```python
from build123d import *

# Parameters (mm, degrees)
BOSS_EXTRUDE1_DEPTH      = 5
BOSS_EXTRUDE1_DEPTH_BACK = 13
SKETCH2_R                = 1.5
CUT_EXTRUDE1_DEPTH       = 66.915554427
SKETCH4_W                = 8
SKETCH4_H                = 4.7
BOSS_EXTRUDE2_DEPTH      = 6
CUT_EXTRUDE3_START       = -5
CUT_EXTRUDE3_DEPTH       = 61.915554427
CUT_EXTRUDE4_DEPTH       = 68.080998169
CHAMFER1_SIZE            = 2.5


with BuildPart() as part:
    # Sketch1 → Boss-Extrude1 (new, two sides: drawn at the far end of the back side and taken through both)
    with BuildSketch(Plane.XY.offset(-BOSS_EXTRUDE1_DEPTH_BACK)):
        Polygon((0, 6), (5, 6), (5, -5), (-20.67950334, -22.556349186), (-49.056349186, -22.556349186), (-60.556349186, -11.056349186), (-46.414213562, 3.085786438), (-34.328427125, -9), (-21.164213562, -9), (-8, 0), (0, 0), align=None)
    extrude(amount=BOSS_EXTRUDE1_DEPTH + BOSS_EXTRUDE1_DEPTH_BACK)

    # Sketch2 → Cut-Extrude1 (cut, through all)
    with BuildSketch(Plane(origin=(0, 0, 0), x_dir=(1, 0, 0), z_dir=(0, 1, 0))):
        with Locations(Location((-3, 3.95, 0), (0, 0, 270))):
            Circle(SKETCH2_R)
    extrude(amount=-CUT_EXTRUDE1_DEPTH, mode=Mode.SUBTRACT)

    # Sketch4 → Boss-Extrude2 (add)
    with BuildSketch(Plane(origin=(0, 0, 0), x_dir=(1, 0, 0), z_dir=(0, 1, 0))):
        with Locations((-4, -2.65)):
            Rectangle(SKETCH4_W, SKETCH4_H)
        with Locations((-4, 10.65)):
            Rectangle(SKETCH4_W, SKETCH4_H)
    extrude(amount=BOSS_EXTRUDE2_DEPTH)

    # Sketch5 → Cut-Extrude3 (cut, through all)
    with BuildSketch(Plane(origin=(0, 0, 0), x_dir=(1, 0, 0), z_dir=(0, 1, 0)).offset(CUT_EXTRUDE3_START)):
        Polygon((-1.267949192, 0.95), (-4.732050808, 0.95), (-6.464101615, 3.95), (-4.732050808, 6.95), (-1.267949192, 6.95), (0.464101615, 3.95), align=None)
    extrude(amount=-CUT_EXTRUDE3_DEPTH, mode=Mode.SUBTRACT)

    # Sketch6 → Cut-Extrude4 (cut, through all)
    with BuildSketch(Plane.XY.offset(5)):
        Polygon((-42.85, -22.556349186), (-49.056349186, -22.556349186), (-60.556349186, -11.056349186), (-46.414213562, 3.085786438), (-34.328427125, -9), (-42.85, -9), align=None)
    extrude(amount=-CUT_EXTRUDE4_DEPTH, mode=Mode.SUBTRACT)

    # Sketch7 → Cut-Revolve1 (revolve, cut)
    with BuildSketch(Plane.XY.offset(-3.95), mode=Mode.PRIVATE) as cut_revolve1_sk:
        Polygon((-24.85, -15.1), (-25.85, -15.1), (-45.997007673, -15.1), (-45.997007673, -12), (-39.790264322, -12), (-38.290264322, -12.35), (-25.85, -12.35), (-24.85, -12.85), align=None)
    revolve(cut_revolve1_sk.sketch.rotate(Axis((-45.997007673, -15.1, -3.95), (1, 0, 0)), 180), axis=Axis((-45.997007673, -15.1, -3.95), (1, 0, 0)), mode=Mode.SUBTRACT)

    # Chamfer1
    chamfer1_edges = [part.edges().sort_by_distance(p)[0] for p in [
        (-42.85, -9, -4),
    ]]
    chamfer(chamfer1_edges, length=CHAMFER1_SIZE)


solid = part.part
```
The model under review builds one solid part; all positions refer to its coordinate system, in mm. A direction names the side the tool comes from. Round coordinates to 2 decimals unless told otherwise and drop trailing zeros. Loops run counter-clockwise (first coordinate to the right, second up) from the corner with the lowest first, then second, coordinate; pieces in that order, holes last. Notation, with made-up numbers: M -14.5,27.5 L 16.5,27.5 A23 cw 16.5,42.5 Z; hole C 13,4 d2. An arc over 180 degrees is marked long. Put each result on its own line as item: value.
Q1. To check wall thickness, follow L1, parallel to Z at x = -41.4, y = -15.1; L2, parallel to Z at x = -1, y = 0.25; L3, parallel to Y at x = -39.5, z = 2.25. State the ranges of each line that lie inside material, in increasing order.
Result set:
L1: z = -13 to -7.05, -0.85 to 5
L2: z = -13 to -8.3, 0.3 to 5
L3: y = -22.56 to -9
Q2. Mouldability with a two-part tool opening along Y and no side actions: class faces 6 (the cylindrical face through (-41.3, -12.82, -6.05)), 7 (the flat face through (-5, 0, -4)), 8 (the flat face through (-5.586, -8.864, -2.429)), 9 (the cylindrical face through (-31.98, -17.64, -2.9)) as released by +Y, released by -Y, zero draft, split by the parting line, or undercut.
Result set:
face 6: undercut
face 7: released by +Y
face 8: zero draft
face 9: undercut
Q3. Consider section C-C, the plane y = -15.1. Give the boundary of the cut face in (x, z).
Result set:
outline: M -42.85,-13 L -9.77,-13 L -9.77,5 L -42.85,5 L -42.85,-0.85 L -39.79,-0.85 L -38.29,-1.2 L -25.85,-1.2 L -24.85,-1.7 L -24.85,-6.2 L -25.85,-6.7 L -38.29,-6.7 L -39.79,-7.05 L -42.85,-7.05 Z
Q4. For pin 1 (3 mm diameter, centred on x = -6, z = 3, fed in from -Y); pin 2 (3 mm diameter, centred on x = -30.5, z = -8.5, fed in from +Y); pin 3 (2.5 mm diameter, centred on x = -3, z = -3.95, fed in from -Y); pin 4 (3 mm diameter, centred on x = -1.5, z = -4, fed in from -Y), all flat-tipped, find the tip position at first contact; note any pin that passes through.
Result set:
pin 1: stops at y = -13.55
pin 2: stops at y = -9
pin 3: passes through
pin 4: stops at y = -5
Q5. Consider section B-B, the plane x = -3. Give the boundary of the cut face in (y, z).
Result set:
outline: M -10.47,-13 L 6,-13 L 6,-8.3 L 0,-8.3 L 0,-5.45 L -5,-5.45 L -5,-6.95 L -10.47,-6.95 Z; M -10.47,-0.95 L -5,-0.95 L -5,-2.45 L 0,-2.45 L 0,0.3 L 6,0.3 L 6,5 L -10.47,5 Z
Q6. Consider section D-D, the plane z = -10.5. Give the boundary of the cut face in (x, y), then the cut area to 3 significant figures.
Result set:
outline: M -42.85,-22.56 L -20.68,-22.56 L 5,-5 L 5,6 L -8,6 L -8,0 L -21.16,-9 L -40.35,-9 L -42.85,-11.5 Z
area: 674 mm²
Q7. Machinability: for faces 1 (the flat face through (1, 6, -4)), 2 (the flat face through (-0.414, -6.636, -5.471)), 3 (the flat face through (-24.85, -15, -4)), 4 (the flat face through (-4, 3, 0.3)), 5 (the flat face through (-8, 3, 3)), which of the approach directions +Z, -Z, +X, -X, +Y, -Y give a long, thin tool a straight path to every point of the face, cutting with its end or side? Answer none if there is none.
Result set:
face 1: +Z, -Z, +X, -X, +Y
face 2: -Y
face 3: -X
face 4: -X, +Y
face 5: +Z, -Z, -X, +Y
Q8. Consider section A-A, the plane z = -0.25. Give the boundary of the cut face in (x, y).
Result set:
outline: M -42.85,-22.56 L -20.68,-22.56 L 5,-5 L 5,6 L 0,6 L 0,0 L -8,0 L -21.16,-9 L -40.35,-9 L -42.85,-11.5 Z
